Can you work these out from the drawing? Everything is in mm from the part's minimum corner. A direction names the side the tool comes from. Give positions to 0.01 mm unless a question says otherwise; leave off trailing zeros. Write each loop counter-clockwise with the first axis right and the second up, starting at its lowest first coordinate (ties: lowest second). Pieces come first, ordered by that corner, then holes. Notation, with made-up numbers: (28.25, -17.5) - (72.25, -17.5) arc R32 ccw to (72.25, 14.5) - close; hole circle Ø10 at (-25, -10.75). An arc over 180 degrees is marked (long way). Use a Markdown table: item, result. Add a question column.
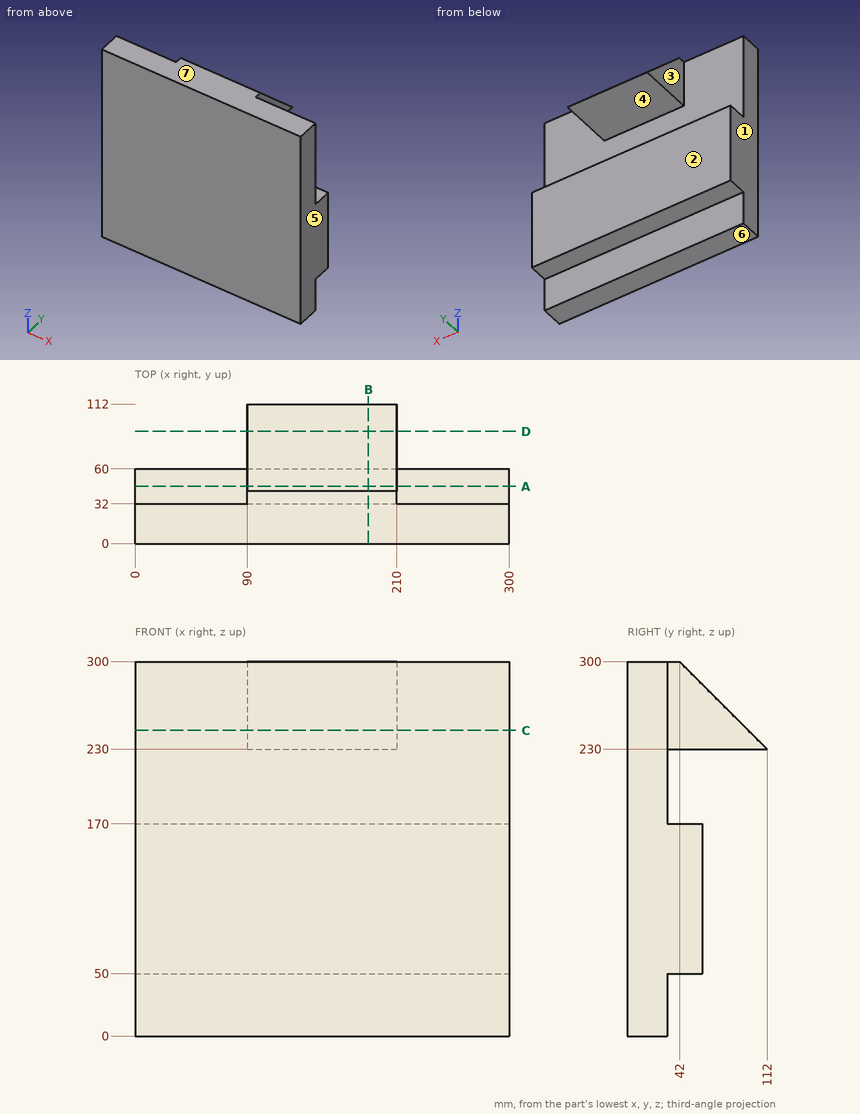
Q1. Suppose I cut it at D-D (y = 90). Please give me the cut outline in (x, z), and give its area (3 significant figures).
Q2. I'm going to push flat-ended pins straight in: P1, Ø5, axis at y = 57, z = 244.5, coming from the -X side; P2, Ø1, axis at x = 133, z = 145.5, coming from the +Y side; P3, Ø3, axis at x = 107.5, z = 173.5, coming from the +Y side. Where does each tip first touch, or does it pass through?
Q3. On a 3-axis mill with a long thin cutter (end or side, diameter ignored), from which of +Z, -Z, +X, -X, +Y, -Y can I reach the whole of each face in a straight line? I mean the marked faces 1, 2 and 3. Say none if no direction works.
Q4. Suppose I cut it at B-B (x = 187). Please give me the cut outline in (y, z), and give its area (3 significant figures).
Q5. Suppose I cut it at A-A (y = 46). Please give me the cut outline in (x, z), and give its area (3 significant figures).
Q6. If we mould it in two halves opening along Z, with no side actions, what happens to the marked faces 4, 5, 6 and 7? For each: released by +Z, released by -Z, zero draft, split by the parting line, or undercut.
Q7. If I drill on probe 1 along Y at (x, z) = (180, 73); probe 2 along Y at (x, z) = (140.5, 35); probe 3 along Z at (x, y) = (232.5, 36), over which ranges is the centre line in solid material (lowest first)? Write a range as [from, to].
Q8. Suppose I cut it at C-C (z = 245). Please give me the cut outline in (x, y).
Derived:
| question | item | result |
|---|---|---|
| 1 | outline | (90, 230) - (210, 230) - (210, 252) - (90, 252) - close |
| 1 | area | 2,640 mm² |
| 2 | P1 | x = 90 |
| 2 | P2 | y = 60 |
| 2 | P3 | y = 32 |
| 3 | face 1 | +Z, -Z, -X, +Y, -Y |
| 3 | face 2 | -Z, +X, -X, +Y |
| 3 | face 3 | +Z, -X, +Y |
| 4 | outline | (0, 0) - (32, 0) - (32, 50) - (60, 50) - (60, 170) - (32, 170) - (32, 230) - (112, 230) - (42, 300) - (0, 300) - close |
| 4 | area | 16,100 mm² |
| 5 | outline | (0, 50) - (300, 50) - (300, 170) - (0, 170) - close; (90, 230) - (210, 230) - (210, 296) - (90, 296) - close |
| 5 | area | 43,900 mm² |
| 6 | face 4 | undercut |
| 6 | face 5 | zero draft |
| 6 | face 6 | released by -Z |
| 6 | face 7 | released by +Z |
| 7 | probe 1 | [0, 60] |
| 7 | probe 2 | [0, 32] |
| 7 | probe 3 | [50, 170] |
| 8 | outline | (0, 0) - (300, 0) - (300, 32) - (210, 32) - (210, 97) - (90, 97) - (90, 32) - (0, 32) - close |
